Can you work these out from the model? Positions are in its coordinate system, mm. A direction names the side the tool comes from. Give positions to 0.01 mm unless a question says otherwise; leave off trailing zeros. Loops run counter-clockwise (first coordinate to the right, second up) from the corner with the lowest first, then second, coordinate; pieces in that order, holes last. Notation, with made-up numbers: (-15, 1) - (28, 1) arc R25 ccw to (28, 36) - close; hole circle Ø7 at (-9, 39.25). An arc over 180 degrees is marked (long way). Answer in a Markdown table with one row per item.
Autodesk Inventor part; units mm, degrees
ref_plane "YZ Plane" through (0, 0, 0) normal (1, 0, 0) x (0, 1, 0)
ref_plane "XZ Plane" through (0, 0, 0) normal (0, 1, 0) x (-1, 0, 0)
ref_plane "XY Plane" through (0, 0, 0) normal (0, 0, 1) x (1, 0, 0)
sketch "Sketch1" plane through (0, 0, 0) normal (0, 1, 0) x (-1, 0, 0)
  line L0 (21.5, 24.5) -> (-21.5, 24.5)
  line L1 (-21.5, 24.5) -> (-21.5, -24.5)
  line L2 (-21.5, -24.5) -> (21.5, -24.5)
  line L3 (21.5, -24.5) -> (21.5, 24.5)
  line L4 (21.5, 24.5) -> (-21.5, -24.5) construction
  line L5 (-21.5, 24.5) -> (21.5, -24.5) construction
  point P0 (0, 0)
  dimension "d0" = 43
  dimension "d1" = 49
extrude "Extrusion1" add sketch "Sketch1" against normal blind 2
sketch "Sketch2" plane through (0, -2, 0) normal (0, -1, 0) x (1, 0, 0)
  line L0 (21.5, -24.5) -> (21.5, 24.5)
  line L1 (21.5, 24.5) -> (-21.5, 24.5)
  line L2 (-21.5, 24.5) -> (-21.5, -24.5)
  line L3 (-21.5, -24.5) -> (21.5, -24.5)
  line L4 (-21.5, 24.5) -> (-18.2, 24.5)
  line L5 (-18.2, 24.5) -> (-18.2, -24.5)
  line L6 (-18.2, -24.5) -> (-21.5, -24.5)
  line L7 (-21.5, -24.5) -> (-21.5, 24.5)
  line L8 (21.5, 24.5) -> (18.2, 24.5)
  line L9 (18.2, 24.5) -> (18.2, -24.5)
  line L10 (18.2, -24.5) -> (21.5, -24.5)
  line L11 (21.5, -24.5) -> (21.5, 24.5)
  line L12 (-18.2, 24.5) -> (18.2, 24.5)
  line L13 (18.2, 24.5) -> (18.2, 16)
  line L14 (18.2, 16) -> (-18.2, 16)
  line L15 (-18.2, 16) -> (-18.2, 24.5)
  line L16 (18.2, -24.5) -> (-18.2, -24.5)
  line L17 (-18.2, -24.5) -> (-18.2, -20.9)
  line L18 (-18.2, -20.9) -> (18.2, -20.9)
  line L19 (18.2, -20.9) -> (18.2, -24.5)
  point P0 (0, 0)
  point P1 (-18.2, 16)
  point P2 (18.2, -20.9)
  dimension "d4" = 3.3
  dimension "d5" = 3.3
  dimension "d6" = 8.5
  dimension "d7" = 3.6
extrude "Extrusion2" add sketch "Sketch2" along normal blind 29.4 contours L3 L9 L1 L0 | L3 L5 L18 L9 | L9 L14 L5 L1 | L3 L2 L1 L5
sketch "Sketch3" plane through (-21.5, 0, 24.5) normal (0, 0, 1) x (1, 0, 0)
  line L0 (0, 0) -> (43, 0)
  line L1 (0, 0) -> (0, -31.4)
  line L2 (43, -31.4) -> (0, -31.4)
  line L3 (43, 0) -> (43, -31.4)
  line L4 (10.7, -31.4) -> (32.3, -31.4)
  line L5 (32.3, -31.4) -> (32.3, -5.6)
  line L6 (32.3, -5.6) -> (10.7, -5.6)
  line L7 (10.7, -5.6) -> (10.7, -31.4)
  point P0 (21.5, 0)
  point P1 (21.5, -31.4)
  dimension "d12" = 21.6
  dimension "d13" = 25.8
  dimension "d14" = 10.8
extrude "Extrusion3" cut sketch "Sketch3" along normal blind 10 from surface at -49 contours L7 L6 L5 L2
fillet "Fillet1" radius 2 4 edges at (21.5, -15.7, 24.5) (21.5, -15.7, -24.5) (-21.5, -15.7, 24.5) (-21.5, -15.7, -24.5)
properties part number "encloser_valve-solenoid" material "ABS Plastic"
Q1. Imagine slicing it at B-B, the plane y = -4. Write out the boundary of the cut face in (x, z), and give its area (3 significant figures).
Checked values:
| item | result |
|---|---|
| outline | (-21.5, -22.5) arc R2 ccw to (-19.5, -24.5) - (19.5, -24.5) arc R2 ccw to (21.5, -22.5) - (21.5, 22.5) arc R2 ccw to (19.5, 24.5) - (-19.5, 24.5) arc R2 ccw to (-21.5, 22.5) - close; hole (-18.2, -20.9) - (18.2, -20.9) - (18.2, 16) - (-18.2, 16) - close |
| area | 760 mm² |
Q2. On a 3-axis mill with a long thin cutter (end or side, diameter ignored), from which of +Z, -Z, +X, -X, +Y, -Y can I reach the whole of each face in a straight line? I mean faces 1 (the face through (-20.93, -15.92, -23.9)), 2 (the face through (18.2, -16, -2)), 3 (the face through (0, -5.6, -23)). Say none if no direction works.
Checked values:
| item | result |
|---|---|
| face 1 | -Z, -X, +Y, -Y |
| face 2 | -Y |
| face 3 | -Z, -Y |
Q3. Imagine slicing it at A-A, the plane x = -10. Write out the boundary of the cut face in (y, z).
Checked values:
| item | result |
|---|---|
| outline | (-31.4, 16) - (-2, 16) - (-2, -20.9) - (-5.6, -20.9) - (-5.6, -24.5) - (0, -24.5) - (0, 24.5) - (-31.4, 24.5) - close |
Q4. If we mould it in two halves opening along X, with no side actions, what happens to faces 4 (the face through (-20.93, -15.48, 23.9)), 5 (the face through (10.8, -19, -23)), 6 (the face through (20.9, -15.48, 23.93))? For each: released by +X, released by -X, zero draft, split by the parting line, or undercut.
Checked values:
| item | result |
|---|---|
| face 4 | released by -X |
| face 5 | undercut |
| face 6 | released by +X |
Q5. Imagine slicing it at C-C, the plane z = 6. Write out the boundary of the cut face in (x, y).
Checked values:
| item | result |
|---|---|
| outline | (-21.5, -31.4) - (-18.2, -31.4) - (-18.2, -2) - (18.2, -2) - (18.2, -31.4) - (21.5, -31.4) - (21.5, 0) - (-21.5, 0) - close |
Q6. If I drill on line 1 (X direction, y = -29.5, z = -17); line 2 (Z direction, x = -11, y = -27.5); line 3 (Y direction, x = 0, z = -21.5), over which ranges is the centre line in solid material (lowest first)? Write a range as [from, to].
Checked values:
| item | result |
|---|---|
| line 1 | x = [-21.5, -18.2], [18.2, 21.5] |
| line 2 | z = [-24.5, -20.9], [16, 24.5] |
| line 3 | y = [-5.6, 0] |
Q7. For pin 1 (2 mm diameter, centred on x = -1.5, y = -12.5, fed in from -Z); pin 2 (2 mm diameter, centred on x = -3, z = 4.5, fed in from -Y); pin 3 (4 mm diameter, centred on x = -3, z = -23, fed in from -Y), each with a flat end and sliding along its axis, tell me the tip position at first contact or that it passes through.
Checked values:
| item | result |
|---|---|
| pin 1 | stops at z = 16 |
| pin 2 | stops at y = -2 |
| pin 3 | stops at y = -5.6 |
Q8. Imagine slicing it at D-D, the plane y = -22. Write out the boundary of the cut face in (x, z), and give its area (3 significant figures).
Checked values:
| item | result |
|---|---|
| outline | (-21.5, -22.5) arc R2 ccw to (-19.5, -24.5) - (-10.8, -24.5) - (-10.8, -20.9) - (-18.2, -20.9) - (-18.2, 16) - (18.2, 16) - (18.2, -20.9) - (10.8, -20.9) - (10.8, -24.5) - (19.5, -24.5) arc R2 ccw to (21.5, -22.5) - (21.5, 22.5) arc R2 ccw to (19.5, 24.5) - (-19.5, 24.5) arc R2 ccw to (-21.5, 22.5) - close |
| area | 683 mm² |
